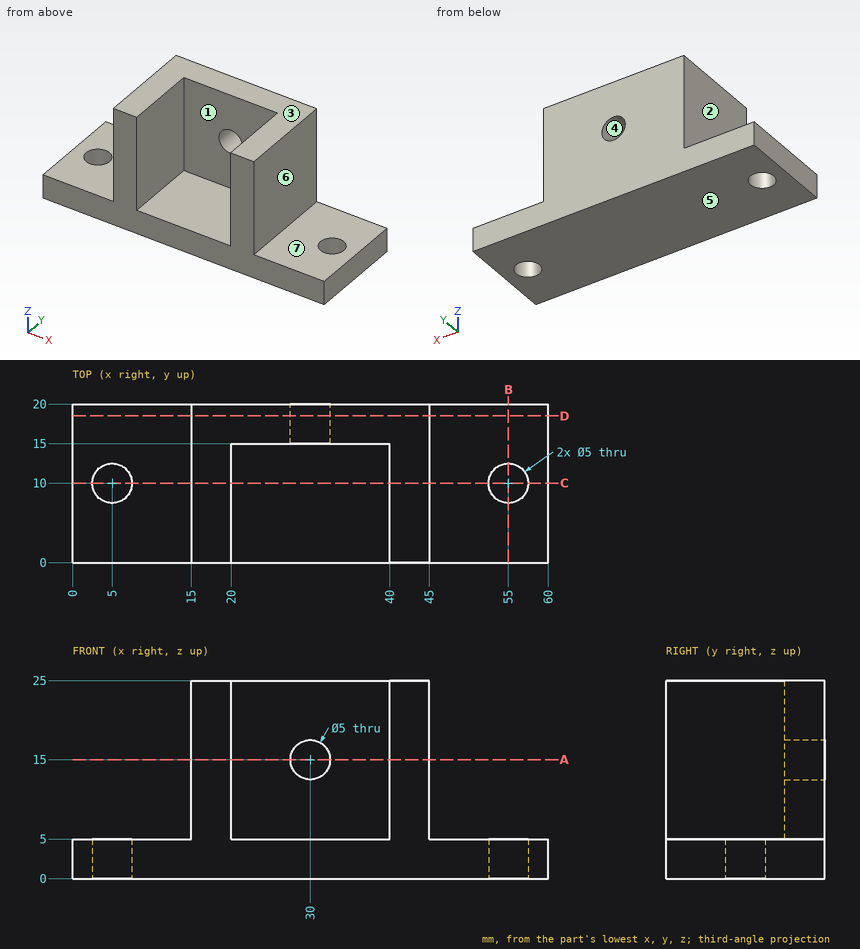
Study the drawing (mm; zero at the part's minimum x, y, z) and answer. A direction names the side the tool comes from. Coordinates: 2 decimals unless noted, no trailing zeros. Write each loop counter-clockwise with the first axis right and the second up, starting at its lowest first coordinate (ties: lowest second). Pieces come first, ordered by that corner, then holes. Notation, with made-up numbers: (39, 86) - (52, 86) arc R14 cw to (52, 97) - close; hole circle Ø11 at (82.25, 73.5). An arc over 180 degrees is marked (long way). Put each result on its own line as item: value.
1. The part is cut by section B-B on x = 55. Give the vertices of the cut face in (y, z).
Answer sheet:
outline: (0, 0) - (7.5, 0) - (7.5, 5) - (0, 5) - close; (12.5, 0) - (20, 0) - (20, 5) - (12.5, 5) - close
2. The part is cut by section D-D on y = 18.5. Give the vertices of the cut face in (x, z), plus the area to 3 significant figures.
Answer sheet:
outline: (0, 0) - (60, 0) - (60, 5) - (45, 5) - (45, 25) - (15, 25) - (15, 5) - (0, 5) - close; hole circle Ø5 at (30, 15)
area: 880 mm^2
3. The part is cut by section C-C on y = 10. Give the vertices of the cut face in (x, z), plus the area to 3 significant figures.
Answer sheet:
outline: (0, 0) - (2.5, 0) - (2.5, 5) - (0, 5) - close; (7.5, 0) - (52.5, 0) - (52.5, 5) - (45, 5) - (45, 25) - (40, 25) - (40, 5) - (20, 5) - (20, 25) - (15, 25) - (15, 5) - (7.5, 5) - close; (57.5, 0) - (60, 0) - (60, 5) - (57.5, 5) - close
area: 450 mm^2
4. Flat-ended cylindrical pins translate along their axes: pin 1 Ø7.5 at (y, z) = (11, 10.5) entering from +X; pin 2 Ø6 at (x, z) = (30, 15) entering from -Y; pin 3 Ø12 at (x, y) = (53, 11.5) entering from +Z; pin 4 Ø5 at (x, y) = (9.5, 7) entering from -Z. Find the tip coordinate at first contact, or state that the pin passes through.
Answer sheet:
pin 1: stops at x = 45
pin 2: stops at y = 15
pin 3: stops at z = 5
pin 4: stops at z = 0
5. Determine the mould class of the marked faces 4, 5, 6 and 7 for opening direction Z: pulls with the +Z half, pulls with the -Z half, needs draft (parallel to the pull), parting line crosses it, or undercut.
Answer sheet:
face 4: undercut
face 5: pulls with the -Z half
face 6: needs draft
face 7: pulls with the +Z half
6. A tool of negligible diameter and unlimited length cuts with its end or side. For the marked faces 1, 2 and 3, from which of +Z, -Z, +X, -X, +Y, -Y can it reach the whole face along a straight path? Write none if from no direction.
Answer sheet:
face 1: +Z, -Y
face 2: +Z, -X, +Y, -Y
face 3: +Z, +X, -X, +Y, -Y
7. The part is cut by section A-A on z = 15. Give the vertices of the cut face in (x, y).
Answer sheet:
outline: (15, 0) - (20, 0) - (20, 15) - (27.5, 15) - (27.5, 20) - (15, 20) - close; (32.5, 15) - (40, 15) - (40, 0) - (45, 0) - (45, 20) - (32.5, 20) - close
8. Find the intervals of material crossed by line 1 along Y through (x, z) = (55, 3.65); line 2 along X through (y, z) = (2.75, 9.25); line 3 along Z through (x, y) = (30, 18.45), in increasing order. Write a range as from..to.
Answer sheet:
line 1: y = 0..7.5, 12.5..20
line 2: x = 15..20, 40..45
line 3: z = 0..12.5, 17.5..25
